from build123d import *

# Parameters (mm, degrees)
BOSS_EXTRUDE1_DEPTH                                 = 70
BOSS_EXTRUDE2_REACH                                 = 115.806
BOSS_EXTRUDE2_START_RADIUS                          = 57
BOSS_EXTRUDE2_END_RADIUS                            = 57
SKETCH7_W                                           = 3
SKETCH7_H                                           = 10
CSK_FOR_M4_COUNTERSUNK_FLAT_HEAD_SCREW2_D           = 4.5
CSK_FOR_M4_COUNTERSUNK_FLAT_HEAD_SCREW2_DEPTH       = 11.5
CSK_FOR_M4_COUNTERSUNK_FLAT_HEAD_SCREW2_CSINK_D     = 9.4
CSK_FOR_M4_COUNTERSUNK_FLAT_HEAD_SCREW2_CSINK_ANGLE = 90
CSK_FOR_M4_COUNTERSUNK_FLAT_HEAD_SCREW2_TIP         = 1.351936393


with BuildPart() as part:
    # Sketch2 → Boss-Extrude1 (new, symmetric)
    with BuildSketch(Plane(origin=(0, 0, 0), x_dir=(1, 0, 0), z_dir=(0, 1, 0))):
        with BuildLine():
            Line((-47.704446333, -36.390737834), (-45.562994128, -34.249285629))
            ThreePointArc((-45.562994128, -34.249285629), (0, -57), (45.562994128, -34.249285629))
            Line((45.562994128, -34.249285629), (47.704446333, -36.390737834))
            ThreePointArc((47.704446333, -36.390737834), (0, -60), (-47.704446333, -36.390737834))
        make_face()
    extrude(amount=BOSS_EXTRUDE1_DEPTH, both=True)

    # Boss-Extrude2: from a cylinder face, 115.806 long prism both ways, kept between that surface and its translate by the depth
    boss_extrude2_start = Plane(origin=(0, 0.207736, 0), z_dir=(0, -1, 0)) * Cylinder(BOSS_EXTRUDE2_START_RADIUS, 477.027472, mode=Mode.PRIVATE)
    boss_extrude2_end = Plane(origin=(0, 0.207736, -10), z_dir=(0, -1, 0)) * Cylinder(BOSS_EXTRUDE2_END_RADIUS, 477.027472, mode=Mode.PRIVATE)
    # Sketch7 → Boss-Extrude2 (add, from a surface)
    with BuildSketch(Plane.XY, mode=Mode.PRIVATE) as boss_extrude2_sk1:
        with Locations((4.5, -65)):
            Rectangle(SKETCH7_W, SKETCH7_H)
    boss_extrude2_tool1 = extrude(boss_extrude2_sk1.sketch, amount=BOSS_EXTRUDE2_REACH, both=True, mode=Mode.PRIVATE)
    add(((boss_extrude2_tool1 & boss_extrude2_start) - boss_extrude2_end).solids().sort_by_distance((4.5, -65, 51.802164))[0])
    # Sketch7 → Boss-Extrude2 (add, from a surface)
    with BuildSketch(Plane.XY, mode=Mode.PRIVATE) as boss_extrude2_sk2:
        with BuildLine():
            Line((3, 65.553629026), (3, 64))
            Line((3, 64), (6, 64))
            Line((6, 64), (6, 67.370437785))
            Line((6, 67.370437785), (3.649292783, 66.490114182))
            ThreePointArc((3.649292783, 66.490114182), (3.178200993, 66.123406518), (3, 65.553629026))
        make_face()
    boss_extrude2_tool2 = extrude(boss_extrude2_sk2.sketch, amount=BOSS_EXTRUDE2_REACH, both=True, mode=Mode.PRIVATE)
    add(((boss_extrude2_tool2 & boss_extrude2_start) - boss_extrude2_end).solids().sort_by_distance((4.5, -65, 51.802164))[0])
    # Sketch7 → Boss-Extrude2 (add, from a surface)
    with BuildSketch(Plane.XY, mode=Mode.PRIVATE) as boss_extrude2_sk3:
        with BuildLine():
            Line((-3, 65.553629026), (-3, 64))
            Line((-3, 64), (-6, 64))
            Line((-6, 64), (-6, 67.370437785))
            Line((-6, 67.370437785), (-3.649292783, 66.490114182))
            ThreePointArc((-3.649292783, 66.490114182), (-3.178200993, 66.123406518), (-3, 65.553629026))
        make_face()
    boss_extrude2_tool3 = extrude(boss_extrude2_sk3.sketch, amount=BOSS_EXTRUDE2_REACH, both=True, mode=Mode.PRIVATE)
    add(((boss_extrude2_tool3 & boss_extrude2_start) - boss_extrude2_end).solids().sort_by_distance((4.5, -65, 51.802164))[0])
    # Sketch7 → Boss-Extrude2 (add, from a surface)
    with BuildSketch(Plane.XY, mode=Mode.PRIVATE) as boss_extrude2_sk4:
        with Locations((-4.5, -65)):
            Rectangle(SKETCH7_W, SKETCH7_H)
    boss_extrude2_tool4 = extrude(boss_extrude2_sk4.sketch, amount=BOSS_EXTRUDE2_REACH, both=True, mode=Mode.PRIVATE)
    add(((boss_extrude2_tool4 & boss_extrude2_start) - boss_extrude2_end).solids().sort_by_distance((4.5, -65, 51.802164))[0])

    # CSK for M4 Countersunk Flat Head Screw2
    with Locations(Plane(origin=(0, 55, 60), x_dir=(1, 0, 0), z_dir=(0, 0, 1))):
        with Locations((0, 0), (0, -110)):
            CounterSinkHole(CSK_FOR_M4_COUNTERSUNK_FLAT_HEAD_SCREW2_D / 2, CSK_FOR_M4_COUNTERSUNK_FLAT_HEAD_SCREW2_CSINK_D / 2, depth=CSK_FOR_M4_COUNTERSUNK_FLAT_HEAD_SCREW2_DEPTH, counter_sink_angle=CSK_FOR_M4_COUNTERSUNK_FLAT_HEAD_SCREW2_CSINK_ANGLE)
            with Locations((0, 0, -(CSK_FOR_M4_COUNTERSUNK_FLAT_HEAD_SCREW2_DEPTH + CSK_FOR_M4_COUNTERSUNK_FLAT_HEAD_SCREW2_TIP / 2))):  # 118° drill point
                Cone(0, CSK_FOR_M4_COUNTERSUNK_FLAT_HEAD_SCREW2_D / 2, CSK_FOR_M4_COUNTERSUNK_FLAT_HEAD_SCREW2_TIP, mode=Mode.SUBTRACT)


solid = part.part
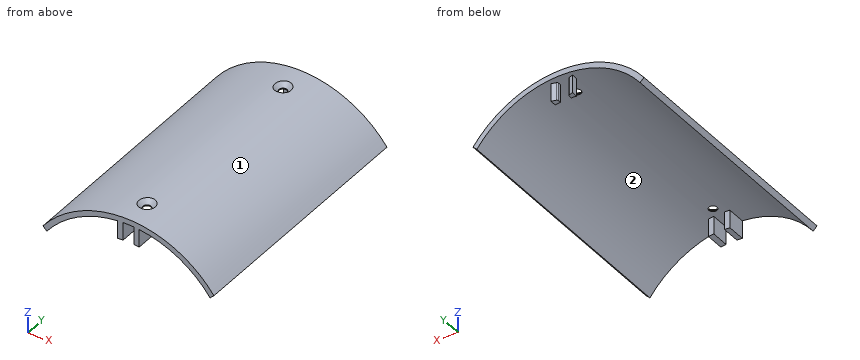
Can you work these out from the model? Positions are in its coordinate system, mm. Face numbers are marked on the shaded views. Coordinates: 2 decimals unless noted, no trailing zeros. Order: outer loops, then holes, each group sorted by start corner. A loop starts at its lowest first (then second) coordinate and runs counter-clockwise, first axis right, second up. Notation, with made-up numbers: M 65,53.5 L 117,53.5 A25 ccw 117,90.5 Z; hole C 72.5,55.25 d8. An arc over 180 degrees is marked long. Answer as CSV lines item,"result".
(1) Suppose I cut it at A-A on x = 0. Please give me the cut outline in (y, z), plus the area to 3 significant figures.
Geometry check:
outline,"M -70,57 L -57.25,57 L -57.25,57.55 L -59.7,60 L -70,60 Z; M -52.75,57 L 52.75,57 L 52.75,57.55 L 50.3,60 L -50.3,60 L -52.75,57.55 Z; M 57.25,57 L 70,57 L 70,60 L 59.7,60 L 57.25,57.55 Z"
area,"381 mm^2"
(2) I'm going to push flat-ended pins straight in: pin 1 (1 mm diameter, centred on y = 1.5, z = 56, fed in from +X); pin 2 (2.5 mm diameter, centred on x = 4, z = 50, fed in from +Y); pin 3 (5 mm diameter, centred on y = 43.5, z = 53, fed in from +X); pin 4 (2.5 mm diameter, centred on x = 0, y = 55, fed in from -Z). Where does each tip first touch, or does it pass through?
Geometry check:
pin 1,"x = 22.8"
pin 2,"y = 67.09"
pin 3,"x = 32.4"
pin 4,"through"
(3) If we mould it in two halves opening along X, with no side actions, what happens to the marked faces 1 and 2? For each: released by +X, released by -X, zero draft, split by the parting line, or undercut.
Geometry check:
face 1,"split by the parting line"
face 2,"undercut"
(4) Please list where these lines run through material, in increasing order: L1, parallel to Y at x = 0, z = 57.4; L2, parallel to X at y = -64, z = 52.75; L3, parallel to Z at x = 6, y = -56.5.
Geometry check:
L1,"-70 to -57.25, -52.75 to 52.75, 57.25 to 70"
L2,"-28.59 to -21.6, -6 to -3, 3 to 6, 21.6 to 28.59"
L3,"56.68 to 59.7"
(5) Suppose I cut it at B-B on z = 39. Please give me the cut outline in (x, y), plus the area to 3 significant figures.
Geometry check:
outline,"M -45.6,-70 L -41.57,-70 L -41.57,70 L -45.6,70 Z; M 41.57,-70 L 45.6,-70 L 45.6,70 L 41.57,70 Z"
area,"1,130 mm^2"
(6) Suppose I cut it at C-C on y = 55. Please give me the cut outline in (x, z).
Geometry check:
outline,"M -47.7,36.39 L -45.56,34.25 A57 cw -2.25,56.96 L -2.25,57.55 L -4.53,59.83 A60 ccw Z; M 2.25,56.96 A57 cw 45.56,34.25 L 47.7,36.39 A60 ccw 4.53,59.83 L 2.25,57.55 Z"
(7) Suppose I cut it at D-D on z = 48.5. Please give me the cut outline in (x, y), plus the area to 3 significant figures.
Geometry check:
outline,"M -35.32,-70 L -29.95,-70 L -29.95,70 L -35.32,70 Z; M -6,-70 L -3,-70 L -3,-60 L -6,-60 Z; M -6,64 L -3,64 L -3,65.55 A1 ccw -3.65,66.49 L -6,67.37 Z; M 3,-70 L 6,-70 L 6,-60 L 3,-60 Z; M 3,64 L 6,64 L 6,67.37 L 3.65,66.49 A1 ccw 3,65.55 Z; M 29.95,-70 L 35.32,-70 L 35.32,70 L 29.95,70 Z"
area,"1,580 mm^2"
